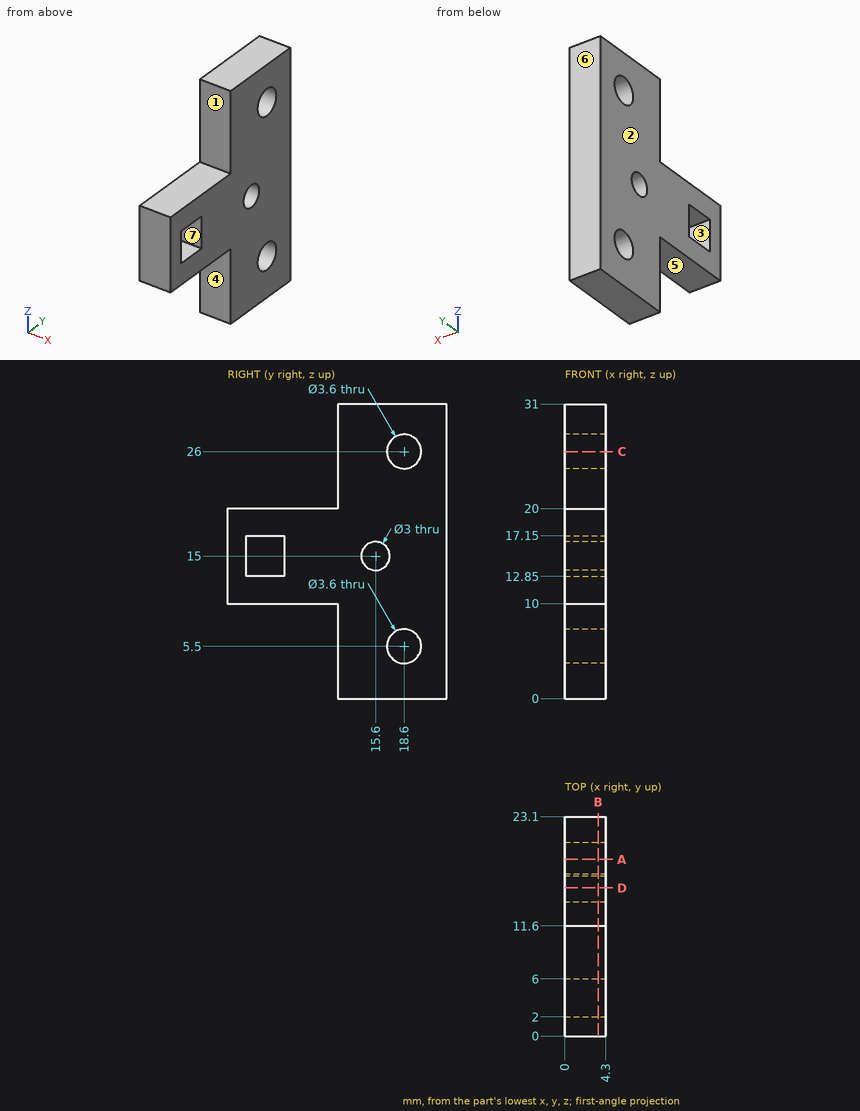
For this review, use the dimensioned drawing (mm, ordinates from the lowest corner) and the shaded views. A direction names the side the tool comes from. Coordinates: 2 decimals unless noted, no trailing zeros. Loops run counter-clockwise (first coordinate to the right, second up) from the corner with the lowest first, then second, coordinate; pieces in that order, holes last. Notation, with made-up numbers: (85, 18.5) -> (90, 18.5) arc R9 ccw to (90, 29.5) -> close; hole circle Ø9 at (29.25, 23). An arc over 180 degrees is marked (long way). Use a Markdown table: item, result. Add a question column.
Item 1: The part is to be moulded in two halves that separate along Z. For the marked faces 5, 6 and 7, say which applies: +Z half, -Z half, draft (parallel to the pull), parting line (faces both ways), or undercut.
Item 2: Machinability: for the marked faces 1, 2, 3 and 4, which of the approach directions +Z, -Z, +X, -X, +Y, -Y give a long, thin tool a straight path to every point of the face, cutting with its end or side? Answer none if there is none.
Item 3: We need section C-C, the plane z = 26. Write out the cut boundary in (x, y), and give its area (3 significant figures).
Item 4: We need section A-A, the plane y = 18.6. Write out the cut boundary in (x, z).
Item 5: Wall thickness on L1, parallel to Z at x = 1.25, y = 18.5; L2, parallel to Z at x = 2.1, y = 15.6; L3, parallel to Z at x = 2.85, y = 20.25: over which ranges is each line inside the solid? List them lowest first. Write a range as from..to.
Item 6: We need section B-B, the plane x = 3.5. Write out the cut boundary in (y, z), and give its area (3 significant figures).
Item 7: We need section D-D, the plane y = 15.6. Write out the cut boundary in (x, z), and give its area (3 significant figures).
Item 8: Clearance check with flat-ended pins moving along their axes: P1, Ø1.3, axis at x = 1.5, y = 5.5, coming from the +Z side; P2, Ø1.2, axis at x = 1.5, y = 4, coming from the -Z side; P3, Ø3, axis at y = 18.6, z = 5.5, coming from the -X side. State where each tip first meets the part, or that it passes through.
Numbers:
| question | item | result |
|---|---|---|
| 1 | face 5 | -Z half |
| 1 | face 6 | draft |
| 1 | face 7 | undercut |
| 2 | face 1 | +Z, +X, -X, -Y |
| 2 | face 2 | +Z, -Z, -X, +Y, -Y |
| 2 | face 3 | +X, -X |
| 2 | face 4 | -Z, +X, -X, -Y |
| 3 | outline | (0, 11.6) -> (4.3, 11.6) -> (4.3, 16.8) -> (0, 16.8) -> close; (0, 20.4) -> (4.3, 20.4) -> (4.3, 23.1) -> (0, 23.1) -> close |
| 3 | area | 34.0 mm^2 |
| 4 | outline | (0, 0) -> (4.3, 0) -> (4.3, 3.7) -> (0, 3.7) -> close; (0, 7.3) -> (4.3, 7.3) -> (4.3, 24.2) -> (0, 24.2) -> close; (0, 27.8) -> (4.3, 27.8) -> (4.3, 31) -> (0, 31) -> close |
| 5 | L1 | z = 0..3.7, 7.3..24.2, 27.8..31 |
| 5 | L2 | z = 0..13.5, 16.5..31 |
| 5 | L3 | z = 0..4.78, 6.22..25.28, 26.72..31 |
| 6 | outline | (0, 10) -> (11.6, 10) -> (11.6, 0) -> (23.1, 0) -> (23.1, 31) -> (11.6, 31) -> (11.6, 20) -> (0, 20) -> close; hole (2, 12.85) -> (6, 12.85) -> (6, 17.15) -> (2, 17.15) -> close; hole circle Ø3 at (15.6, 15); hole circle Ø3.6 at (18.6, 5.5); hole circle Ø3.6 at (18.6, 26) |
| 6 | area | 428 mm^2 |
| 7 | outline | (0, 0) -> (4.3, 0) -> (4.3, 13.5) -> (0, 13.5) -> close; (0, 16.5) -> (4.3, 16.5) -> (4.3, 31) -> (0, 31) -> close |
| 7 | area | 120 mm^2 |
| 8 | P1 | stops at z = 20 |
| 8 | P2 | stops at z = 10 |
| 8 | P3 | passes through |
